Work out the finished part from the listing and answer in its coordinate system (mm). Coordinates: 2 decimals unless noted, no trailing zeros. Write each loop counter-clockwise with the first axis right and the second up, starting at its lowest first coordinate (ties: lowest second). Pieces come first, ordered by that corner, then holes. Notation, with made-up numbers: M 61,27 L 96,27 A22 ccw 96,61 Z; hole C 85.5,62.5 d10. An arc over 180 degrees is marked long. Answer as CSV lines item,"result". Start each with the question number.
(1) A cutting plane is placed at A-A on x = 0.45. Give the vertices of the cut face in (y, z) (3 decimals).
(2) A cutting plane is placed at D-D on y = -5.5. Give the vertices of the cut face in (x, z).
(3) Find the intervals of material crossed by L1, parallel to Y at x = -0.35, z = 0; L2, parallel to Z at x = 0.4, y = 0.25; L3, parallel to Z at x = -0.4, y = -0.5, in increasing order. Write a range as [from, to].
(4) A cutting plane is placed at C-C on z = 29. Give the vertices of the cut face in (x, y), then the cut area to 3 significant figures.
(5) A cutting plane is placed at B-B on y = 0. Give the vertices of the cut face in (x, z), then the cut area to 3 significant figures.
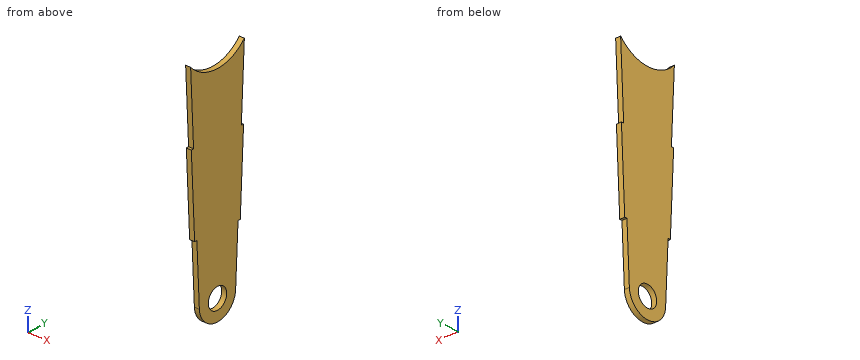
from build123d import *

# Parameters (mm, degrees)
SKETCH1_R           = 3.2639
BOSS_EXTRUDE1_DEPTH = 0.79375


with BuildPart() as part:
    # Sketch1 → Boss-Extrude1 (new, symmetric)
    with BuildSketch(Plane(origin=(0, 0, 0), x_dir=(0, 0, -1), z_dir=(1, 0, 0))):
        with BuildLine():
            Line((-43.495639045, 8.454512603), (-66.675, 9.525))
            ThreePointArc((-66.675, 9.525), (-62.375260413, 0), (-66.675, -9.525))
            Line((-66.675, -9.525), (-44.125906356, -8.483620102))
            Line((-44.125906356, -8.483620102), (-44.089248772, -9.277370102))
            Line((-44.089248772, -9.277370102), (-18.716292707, -8.105576378))
            Line((-18.716292707, -8.105576378), (-18.752950291, -7.311826378))
            Line((-18.752950291, -7.311826378), (0.297049709, -6.432044362))
            ThreePointArc((0.297049709, -6.432044362), (6.4389, 0), (0.297049709, 6.432044362))
            Line((0.297049709, 6.432044362), (-18.12268298, 7.28271888))
            Line((-18.12268298, 7.28271888), (-18.086064426, 8.075623757))
            Line((-18.086064426, 8.075623757), (-43.459020491, 9.24741748))
            Line((-43.459020491, 9.24741748), (-43.495639045, 8.454512603))
        make_face()
        Circle(SKETCH1_R, mode=Mode.SUBTRACT)
    extrude(amount=BOSS_EXTRUDE1_DEPTH, both=True)


solid = part.part
Here are the results:
1,outline,"M -9.525,66.675 L -8.484,44.126 L -9.277,44.089 L -8.106,18.716 L -7.312,18.753 L -6.432,-0.297 A6.439 ccw 6.432,-0.297 L 7.283,18.123 L 8.076,18.086 L 9.247,43.459 L 8.455,43.496 L 9.525,66.675 A12.7 cw Z; hole C 0,0 d6.528"
2,outline,"M -0.79,-3.35 L 0.79,-3.35 L 0.79,63.63 L -0.79,63.63 Z"
3,L1,"y = [-6.45, -3.26], [3.26, 6.45]"
3,L2,"z = [-6.43, -3.25], [3.25, 62.38]"
3,L3,"z = [-6.42, -3.23], [3.23, 62.39]"
4,outline,"M -0.79,-8.58 L 0.79,-8.58 L 0.79,8.58 L -0.79,8.58 Z"
4,area,"27.2 mm^2"
5,outline,"M -0.79,-6.44 L 0.79,-6.44 L 0.79,-3.26 L -0.79,-3.26 Z; M -0.79,3.26 L 0.79,3.26 L 0.79,62.38 L -0.79,62.38 Z"
5,area,"98.9 mm^2"
